CAD build for the part. Positions are in the model's coordinates, mm. A direction names the side the tool comes from. Round coordinates to 2 decimals unless told otherwise and drop trailing zeros. Order: outer loops, then holes, each group sorted by start corner. A loop starts at its lowest first (then second) coordinate and runs counter-clockwise, first axis right, second up. Notation, with made-up numbers: (-25, 71.5) - (3, 71.5) arc R25 ccw to (3, 94.5) - close; hole circle Ø10 at (-12.75, 27.25). An arc over 180 degrees is marked (long way). Use one line per item in the form item = value. Start each with the question number.
from build123d import *

# Parameters (mm, degrees)
RESSALTO_EXTRUS_O1_DEPTH = 17
ESBO_O2_W                = 12
ESBO_O2_H                = 10
RESSALTO_EXTRUS_O2_DEPTH = 9
ESBO_O3_R                = 2
RESSALTO_EXTRUS_O3_DEPTH = 0.7
ESBO_O4_R                = 1.5
RESSALTO_EXTRUS_O4_DEPTH = 9.3
CORTE_EXTRUS_O1_START    = -9.3
CORTE_EXTRUS_O1_DEPTH    = 9.3


with BuildPart() as part:
    # Esboço1 → Ressalto-extrusão1 (new body)
    with BuildSketch(Plane.XY):
        with BuildLine():
            Line((-3.5, 5), (3.5, 5))
            ThreePointArc((3.5, 5), (6.590169944, 0), (3.5, -5))
            Line((3.5, -5), (-3.5, -5))
            ThreePointArc((-3.5, -5), (-6.590169944, 0), (-3.5, 5))
        make_face()
    extrude(amount=-RESSALTO_EXTRUS_O1_DEPTH)

    # Esboço2 → Ressalto-extrusão2 (add)
    with BuildSketch(Plane.XY):
        Rectangle(ESBO_O2_W, ESBO_O2_H)
    extrude(amount=RESSALTO_EXTRUS_O2_DEPTH)

    # Esboço3 → Ressalto-extrusão3 (add)
    with BuildSketch(Plane.XY.offset(9)):
        Circle(ESBO_O3_R)
    extrude(amount=RESSALTO_EXTRUS_O3_DEPTH)

    # Esboço4 → Ressalto-extrusão4 (add)
    with BuildSketch(Plane.XY.offset(9.7)):
        Circle(ESBO_O4_R)
    extrude(amount=RESSALTO_EXTRUS_O4_DEPTH)

    # Esboço5 → Corte-extrusão1 (cut)
    with BuildSketch(Plane.XY.offset(19).offset(CORTE_EXTRUS_O1_START)):
        with BuildLine():
            Line((-1.118033989, 1), (1.118033989, 1))
            ThreePointArc((1.118033989, 1), (0, 1.5), (-1.118033989, 1))
        make_face()
    extrude(amount=CORTE_EXTRUS_O1_DEPTH, mode=Mode.SUBTRACT)


solid = part.part
(1) Slice it at D-D (y = 4). Give the cut face in (x, z), and give its area (3 significant figures).
(2) Flat gauge pins, fed straight in: P1, Ø0.5, axis at x = 6.5, y = 0, coming from the +Z side; P2, Ø6, axis at y = -1, z = -5.5, coming from the -X side; P3, Ø2, axis at y = 2.5, z = 4.5, coming from the +X side; P4, Ø2, axis at x = 0.5, y = 2.5, coming from the +Z side. Where does each tip first touch, or does it go through?
(3) Wall check: line 1 (Z direction, x = -4.75, y = 1); line 2 (X direction, y = -1, z = 3.5); line 3 (Y direction, x = -1, z = 15.5). Give the ranges that are in metal, low to high. Write a range as [from, to].
(4) Slice it at B-B (x = 0). Give the cut face in (y, z), and give its area (3 significant figures).
(5) Slice it at A-A (y = 0). Give the cut face in (x, z), and give its area (3 significant figures).
(6) Slice it at C-C (z = 7.5). Give the cut face in (x, y), and give its area (3 significant figures).
(7) Which spindle directions (+Z, -Z, +X, -X, +Y, -Y) get a long thin tool onto all of the face, cutting with end or side? Do faces 1 (the flat face through (5.3, 4.3, 0)), 2 (the flat face through (-5.3, 4.3, 0)), 3 (the flat face through (0, 1, 14)), 4 (the cylindrical face through (0, -1.5, 14.3)), 5 (the flat face through (5.3, -4.3, 0)). Say none if no direction does.
Results list:
q1.outline = (-6, 0) - (-4.91, 0) - (-4.91, -17) - (4.91, -17) - (4.91, 0) - (6, 0) - (6, 9) - (-6, 9) - close
q1.area = 275 mm²
q2.P1 = 0
q2.P2 = -6.59
q2.P3 = 6
q2.P4 = 9.7
q3.line_1 = [-17, 9]
q3.line_2 = [-6, 6]
q3.line_3 = [-1.12, 1]
q4.outline = (-5, -17) - (5, -17) - (5, 9) - (2, 9) - (2, 9.7) - (1, 9.7) - (1, 19) - (-1.5, 19) - (-1.5, 9.7) - (-2, 9.7) - (-2, 9) - (-5, 9) - close
q4.area = 286 mm²
q5.outline = (-6.59, -17) - (6.59, -17) - (6.59, 0) - (6, 0) - (6, 9) - (2, 9) - (2, 9.7) - (1.5, 9.7) - (1.5, 19) - (-1.5, 19) - (-1.5, 9.7) - (-2, 9.7) - (-2, 9) - (-6, 9) - (-6, 0) - (-6.59, 0) - close
q5.area = 363 mm²
q6.outline = (-6, -5) - (6, -5) - (6, 5) - (-6, 5) - close
q6.area = 120 mm²
q7.face_1 = -Z, +X, +Y
q7.face_2 = -Z, -X, +Y
q7.face_3 = +Z, +X, -X, +Y
q7.face_4 = +Z
q7.face_5 = -Z, +X, -Y
